Build history of the part. All positions in model axes, mm. Face numbers are marked on the shaded views. A direction names the side the tool comes from. Coordinates: 2 decimals unless noted, no trailing zeros. Order: outer loops, then holes, each group sorted by start corner. A loop starts at its lowest first (then second) coordinate and runs counter-clockwise, first axis right, second up. Notation, with made-up numbers: M 83,-39 L 98,-39 A13 ccw 98,-32 Z; hole C 76,70 d9. An arc over 180 degrees is marked long. Write item = value, one per line. Start each with the question number.
Q1. Pin check, flat tips, straight feed: P1, Ø1.5, axis at x = -21, z = 7.5, coming from the +Y side; P2, Ø2, axis at x = -21, z = 15, coming from the -Y side; P3, Ø5, axis at x = 18, z = 25.5, coming from the -Y side; P4, Ø10, axis at y = 139, z = 18, coming from the +X side. Stop position of each tip, or through.
Q2. 3-axis set-ups, long thin cutter, end or side, ignore diameter. For the marked faces 1 and 2: which of +Z, -Z, +X, -X, +Y, -Y reach the whole face in a straight line?
Q3. Band-saw the part on C-C on y = 166.5. Write the cut outline in (x, z).
Q4. Drill centre lines: probe 1 along Z at (x, y) = (-2.5, 138); probe 2 along X at (y, z) = (63, -23); probe 3 along Y at (x, z) = (27.5, -2.5). Where is each one in solid material? Low to high.
```python
from build123d import *

# Parameters (mm, degrees)
SZKIC1_R                    = 25
DODANIE_WYCI_GNI_CIE1_DEPTH = 225
SZKIC2_R                    = 33
DODANIE_WYCI_GNI_CIE2_DEPTH = 18
ZAOKR_GLENIE1_R             = 15
ZAOKR_GLENIE2_R             = 3


with BuildPart() as part:
    # Szkic1 → Dodanie-wyciągnięcie1 (new body)
    with BuildSketch(Plane(origin=(0, 0, 0), x_dir=(1, 0, 0), z_dir=(0, 1, 0))):
        with Locations(Location((0, 0, 0), (0, 0, 270))):
            Circle(SZKIC1_R)
    extrude(amount=DODANIE_WYCI_GNI_CIE1_DEPTH)

    # Szkic2 → Dodanie-wyciągnięcie2 (add)
    with BuildSketch(Plane(origin=(0, 225, 0), x_dir=(1, 0, 0), z_dir=(0, 1, 0))):
        with Locations(Location((0, 0, 0), (0, 0, 270))):
            Circle(SZKIC2_R)
    extrude(amount=DODANIE_WYCI_GNI_CIE2_DEPTH)

    # Zaokrąglenie1
    zaokr_glenie1_edges = [part.edges().sort_by_distance(p)[0] for p in [
        (0, 243, -33),
    ]]
    fillet(zaokr_glenie1_edges, radius=ZAOKR_GLENIE1_R)

    # Zaokrąglenie2
    zaokr_glenie2_edges = [part.edges().sort_by_distance(p)[0] for p in [
        (0, 225, -33),
    ]]
    fillet(zaokr_glenie2_edges, radius=ZAOKR_GLENIE2_R - 0.0001)  # a hair under: the kernel refuses the full size


solid = part.part
```
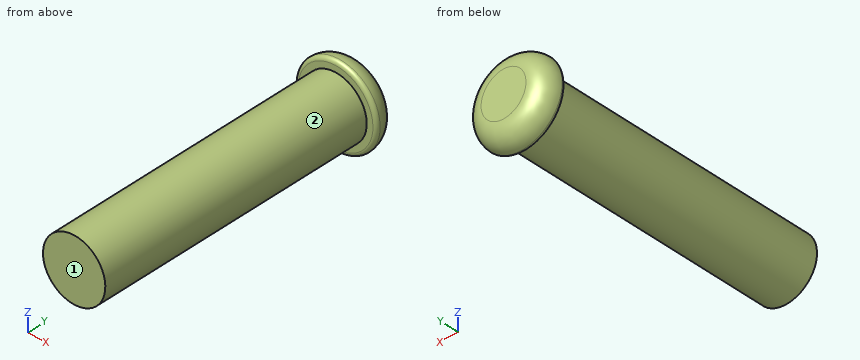
Recorded:
q1.P1 = 242.57
q1.P2 = 0
q1.P3 = 225
q1.P4 = 21.35
q2.face_1 = +Z, -Z, +X, -X, -Y
q2.face_2 = -Y
q3.outline = C 0,0 d50
q4.probe_1 = -24.87 to 24.87
q4.probe_2 = -9.8 to 9.8
q4.probe_3 = 225 to 239.51
